The listing builds one solid part. Answer for the finished solid, in the listing's coordinates (mm). Face numbers are marked on the shaded views. A direction names the side the tool comes from. Round coordinates to 2 decimals unless told otherwise and drop trailing zeros. Write each loop counter-clockwise with the first axis right and the second up, starting at its lowest first coordinate (ties: lowest second). Pieces come first, ordered by that corner, then holes.
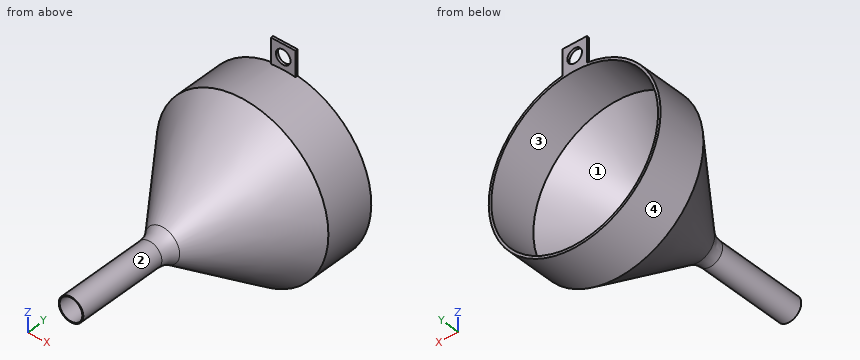
from build123d import *

# Parameters (mm, degrees)
VACIADO1_T              = -2
SALIENTE_EXTRUIR1_DEPTH = 2
CROQUIS3_R              = 5.931653108
CORTAR_EXTRUIR1_DEPTH   = 22
CROQUIS4_R              = 9.206232533
CORTAR_EXTRUIR2_DEPTH   = 82
REDONDEO1_R             = 20


with BuildPart() as part:
    # Croquis1 → Revolución1 (revolve)
    with BuildSketch(Plane.XY, mode=Mode.PRIVATE) as revoluci_n1_sk:
        Polygon((10, -20), (70, 60), (70, 100), (0, 100), (0, -100), (10, -100), align=None)
    revolve(revoluci_n1_sk.sketch.rotate(Axis((0, 100, 0), (0, -1, 0)), 180), axis=Axis((0, 100, 0), (0, -1, 0)))

    # Vaciado1
    vaciado1_openings = [part.faces().sort_by_distance(p)[0] for p in [
        (0, -100, 0),
        (0, 100, 0),
    ]]
    offset(amount=VACIADO1_T, openings=vaciado1_openings, kind=Kind.INTERSECTION)

    # Croquis2 → Saliente-Extruir1 (add)
    with BuildSketch(Plane(origin=(0, 100, 0), x_dir=(1, 0, 0), z_dir=(0, 1, 0))):
        with BuildLine():
            ThreePointArc((10, -69.282032303), (5.012870376, -69.82027736), (0, -70))
            Line((0, -70), (0, -90))
            Line((0, -90), (10, -90))
            Line((10, -90), (10, -69.282032303))
        make_face()
        with BuildLine():
            Line((0, -90), (0, -70))
            ThreePointArc((0, -70), (-5.012870376, -69.82027736), (-10, -69.282032303))
            Line((-10, -69.282032303), (-10, -90))
            Line((-10, -90), (0, -90))
        make_face()
    extrude(amount=-SALIENTE_EXTRUIR1_DEPTH)

    # Croquis3 → Cortar-Extruir1 (cut)
    with BuildSketch(Plane(origin=(0, 100, 0), x_dir=(1, 0, 0), z_dir=(0, 1, 0))):
        with Locations(Location((0, -79.795784901, 0), (0, 0, 180))):
            Circle(CROQUIS3_R)
    extrude(amount=-CORTAR_EXTRUIR1_DEPTH, mode=Mode.SUBTRACT)

    # Croquis4 → Cortar-Extruir2 (cut)
    with BuildSketch(Plane(origin=(0, -100, 0), x_dir=(-1, 0, 0), z_dir=(0, -1, 0))):
        with Locations(Location((0, 0, 0), (0, 0, 180))):
            Circle(CROQUIS4_R)
    extrude(amount=-CORTAR_EXTRUIR2_DEPTH, mode=Mode.SUBTRACT)

    # Redondeo1
    redondeo1_edges = [part.edges().sort_by_distance(p)[0] for p in [
        (10, -20, 0),
    ]]
    fillet(redondeo1_edges, radius=REDONDEO1_R)


solid = part.part
1. Section C-C on y = -36 is taken. Determine the outline of the cut face in (x, z), plus the area to 3 significant figures.
Geometry says:
outline: circle Ø20 at (0, 0); hole circle Ø18.41 at (0, 0)
area: 47.9 mm2
2. Section A-A on y = 79 is taken. Determine the outline of the cut face in (x, z), plus the area to 3 significant figures.
Geometry says:
outline: circle Ø140 at (0, 0); hole circle Ø136 at (0, 0)
area: 867 mm2
3. Given pin 1 (1.5 mm diameter, centred on y = -46.5, z = -6, fed in from +X); pin 2 (8 mm diameter, centred on x = -42, z = 21.5, fed in from +Y); pin 3 (5 mm diameter, centred on y = 30, z = 39, fed in from -X), each flat-ended and moving along its own axis, determine where each tip first touches the part or whether it passes through.
Geometry says:
pin 1: stops at x = 8.51
pin 2: stops at y = 38.24
pin 3: stops at x = -31.59
4. A tool of negligible diameter and unlimited length cuts with its end or side. For the marked faces 1 and 2, from which of +Z, -Z, +X, -X, +Y, -Y can it reach the whole face along a straight path? Write none if from no direction.
Geometry says:
face 1: +Y
face 2: -Y
5. For a pull along X with two mould halves and no side action, classify the marked faces 3 and 4 as released by +X, released by -X, zero draft, split by the parting line, or undercut.
Geometry says:
face 3: undercut
face 4: split by the parting line
6. Straight lines are drawn through the part: line 1 along Z through (x, y) = (0, 99.6); line 2 along Z through (x, y) = (0, 70); line 3 along X through (y, z) = (14, 10.5). For each, find the intervals that lie inside material, in ascending order.
Geometry says:
line 1: z = -70 to -68, 68 to 73.86, 85.73 to 90
line 2: z = -70 to -68, 68 to 70
line 3: x = -33.91 to -31.28, 31.28 to 33.91
7. Section B-B on x = 0 is taken. Give the number of separate pieces and of enclosed holes in the cut face, plus the area to 3 significant figures.
Geometry says:
separate pieces: 3
enclosed holes: 0
area: 709 mm2
